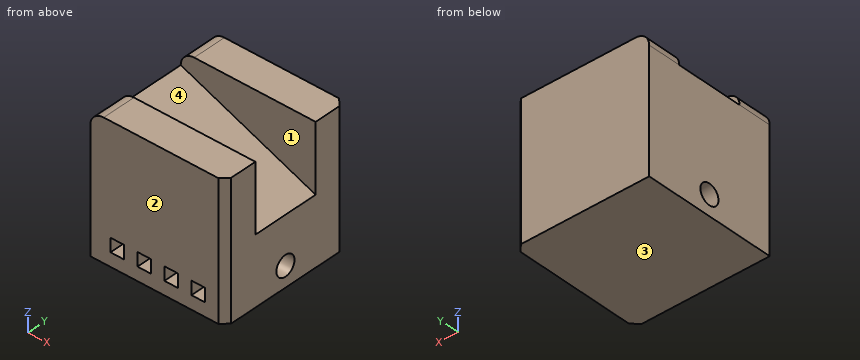
from build123d import *

# Parameters (mm, degrees)
F0_W     = 10
F0_H     = 10
F1_DEPTH = 100
F2_W     = 100
F2_H     = 25
F3_DEPTH = 100
F4_R     = 10
F6_D     = 15
F7_DEPTH = 20
F8_SIZE  = 5


with BuildPart() as f1:
    # F0 (on Front) → F1 (new body)
    with BuildSketch(Plane.XZ):
        Polygon((100, 50), (0, 90), (0, 10), (0, 0), (100, 0), align=None)
        with Locations((20, 15)):
            Rectangle(F0_W, F0_H, mode=Mode.SUBTRACT)
        with Locations((40, 15)):
            Rectangle(F0_W, F0_H, mode=Mode.SUBTRACT)
        with Locations((60, 15)):
            Rectangle(F0_W, F0_H, mode=Mode.SUBTRACT)
        with Locations((80, 15)):
            Rectangle(F0_W, F0_H, mode=Mode.SUBTRACT)
    extrude(amount=-F1_DEPTH)

    # F2 (on face) → F3 (join)
    with BuildSketch(Plane(origin=(0, 0, 0), x_dir=(1, 0, 0), z_dir=(0, 0, -1))):
        with Locations((50, -12.5)):
            Rectangle(F2_W, F2_H)
        with Locations((50, -87.5)):
            Rectangle(F2_W, F2_H)
    extrude(amount=-F3_DEPTH)

    # F4
    f4_edges = [f1.edges().sort_by_distance(p)[0] for p in [
        (0, 12.5, 100),
        (0, 87.5, 100),
    ]]
    fillet(f4_edges, radius=F4_R)

    # F6 (through all)
    with Locations(Plane(origin=(0, 0, 0), x_dir=(0, -1, 0), z_dir=(-1, 0, 0))):
        with Locations((-50, 15)):
            Hole(F6_D / 2)

    # F0 (on Front) → F7 (cut)
    with BuildSketch(Plane.XZ):
        with Locations((80, 15)):
            Rectangle(F0_W, F0_H)
        with Locations((60, 15)):
            Rectangle(F0_W, F0_H)
        with Locations((40, 15)):
            Rectangle(F0_W, F0_H)
        with Locations((20, 15)):
            Rectangle(F0_W, F0_H)
    extrude(amount=-F7_DEPTH, mode=Mode.SUBTRACT)

    # F8
    f8_edges = [f1.edges().sort_by_distance(p)[0] for p in [
        (100, 0, 50),
        (100, 100, 50),
    ]]
    chamfer(f8_edges, length=F8_SIZE)


solid = f1.part
For this review, take the finished solid that the model builds, in its own axes (mm). Face numbers are marked on the shaded views. Give positions to 0.01 mm unless a question says otherwise; leave off trailing zeros. Order: outer loops, then holes, each group sorted by start corner. A loop starts at its lowest first (then second) coordinate and runs counter-clockwise, first axis right, second up. Notation, with made-up numbers: (27.5, 38.25) - (60.5, 38.25) arc R27 ccw to (60.5, 74.25) - close; hole circle Ø8 at (68.25, -28.5). An arc over 180 degrees is marked (long way). Answer as a JSON object with one key per item and string values. Group by question number.
Item 1: Clearance check with flat-ended pins moving along their axes: pin 1 Ø11 at (x, y) = (22, 8.5) entering from -Z; pin 2 Ø8 at (x, y) = (40.5, 32) entering from +Z; pin 3 Ø3 at (x, z) = (58.5, 16) entering from -Y; pin 4 Ø5 at (x, y) = (41, 69.5) entering from +Z. State where each tip first meets the part, or that it passes through.
Item 2: Take a section at D-D on z = 61.5. Give the boundary of the cut face in (x, y).
Item 3: Take a section at C-C on y = 70. Give the boundary of the cut face in (x, z), and give its area (3 significant figures).
Item 4: Draft analysis for pull direction Y (two halves, no side actions). For the marked faces 1, 2, 3 and 4, state which applies: pulls with the +Y half, pulls with the -Y half, needs draft (parallel to the pull), parting line crosses it, or undercut.
Item 5: Wall thickness on line 1 along X through (y, z) = (37.5, 19); line 2 along Y through (x, z) = (50, 15); line 3 along Y through (x, z) = (93, 75.5): over which ranges is each line inside the solid? List them lowest first.
Item 6: Take a section at A-A on y = 50. Give the boundary of the cut face in (x, z).
Item 7: Take a section at B-B on x = 59. Give the boundary of the cut face in (y, z), and give its area (3 significant figures).
Reported:
{
 "1": {"pin 1": "z = 0", "pin 2": "z = 75.4", "pin 3": "y = 20", "pin 4": "z = 74.6"},
 "2": {"outline": "(0, 0) - (95, 0) - (100, 5) - (100, 25) - (71.25, 25) - (71.25, 75) - (100, 75) - (100, 95) - (95, 100) - (0, 100) - close"},
 "3": {"outline": "(0, 0) - (100, 0) - (100, 50) - (0, 90) - close; hole (15, 10) - (25, 10) - (25, 20) - (15, 20) - close; hole (35, 10) - (45, 10) - (45, 20) - (35, 20) - close; hole (55, 10) - (65, 10) - (65, 20) - (55, 20) - close; hole (75, 10) - (85, 10) - (85, 20) - (75, 20) - close", "area": "6,600 mm^2"},
 "4": {"face 1": "undercut", "face 2": "pulls with the -Y half", "face 3": "needs draft", "face 4": "undercut"},
 "5": {"line 1": "0 to 15, 25 to 35, 45 to 55, 65 to 75, 85 to 100", "line 2": "0 to 42.5, 57.5 to 100", "line 3": "0 to 25, 75 to 100"},
 "6": {"outline": "(0, 0) - (100, 0) - (100, 7.5) - (0, 7.5) - close; (0, 22.5) - (100, 22.5) - (100, 50) - (0, 90) - close"},
 "7": {"outline": "(0, 0) - (100, 0) - (100, 100) - (75, 100) - (75, 66.4) - (25, 66.4) - (25, 100) - (0, 100) - (0, 20) - (20, 20) - (20, 10) - (0, 10) - close; hole (25, 10) - (44.41, 10) arc R7.5 ccw to (55.59, 10) - (75, 10) - (75, 20) - (55.59, 20) arc R7.5 ccw to (44.41, 20) - (25, 20) - close", "area": "7,580 mm^2"}
}
